```python
from build123d import *

# Parameters (mm, degrees)
PAD005_DEPTH           = 25
SKETCH014_W            = 3.1
SKETCH014_H            = 3.1
POCKET008_DEPTH        = 3.2
POCKET010_DEPTH        = 20.801
POCKET011_DEPTH        = 0.5
CHAMFER002_SIZE        = 0.5
SKETCH019_R            = 0.75
SKETCH019_R_2          = 1
POCKET012_DEPTH        = 25.001
CHAMFER003_SIZE        = 0.25
PAD009_DEPTH           = 1
CHAMFER_SIZE           = 0.5
PAD021_DEPTH           = 0.5
LINEARPATTERN001_COUNT = 4
LINEARPATTERN001_PITCH = 3.3333333333
SKETCH047_W            = 1.55
SKETCH047_H            = 10.5
PAD022_DEPTH           = 1
SKETCH048_W            = 1.5
SKETCH048_H            = 1.5
PAD023_DEPTH           = 4
SKETCH054_W            = 7.578003
SKETCH054_H            = 26.545825
POCKET038_DEPTH        = 8.751
POCKET038_DEPTH_BACK   = 8.751
FILLET005_R            = 0.5
SKETCH055_W            = 1.5
SKETCH055_H            = 1.5
POCKET039_DEPTH        = 2


with BuildPart() as part:
    # Sketch013 → Pad005 (new body)
    with BuildSketch(Plane.XY):
        with BuildLine():
            Line((-6.75, 4.75), (6.75, 4.75))
            ThreePointArc((8.75, 2.75), (8.1642135624, 4.1642135624), (6.75, 4.75))
            Line((8.75, 2.75), (8.75, -2.75))
            ThreePointArc((6.75, -4.75), (8.1642135624, -4.1642135624), (8.75, -2.75))
            Line((6.75, -4.75), (-6.75, -4.75))
            ThreePointArc((-8.75, -2.75), (-8.1642135624, -4.1642135624), (-6.75, -4.75))
            Line((-8.75, -2.75), (-8.75, 2.75))
            ThreePointArc((-6.75, 4.75), (-8.1642135624, 4.1642135624), (-8.75, 2.75))
        make_face()
    extrude(amount=-PAD005_DEPTH)

    # Sketch014 (on Face9 of Pad005) → Pocket008 (cut)
    with BuildSketch(Plane.XY):
        with Locations((6.15, 0)):
            Rectangle(SKETCH014_W, SKETCH014_H)
        with Locations((-6.15, 0)):
            Rectangle(SKETCH014_W, SKETCH014_H)
    extrude(amount=-POCKET008_DEPTH, mode=Mode.SUBTRACT)

    # Sketch017 → Pocket010 (cut, through all)
    with BuildSketch(Plane.XY.offset(-4.2)):
        with BuildLine():
            Line((-6.75, 3.75), (6.75, 3.75))
            ThreePointArc((7.75, 2.75), (7.4571067812, 3.4571067812), (6.75, 3.75))
            Line((7.75, 2.75), (7.75, -2.75))
            ThreePointArc((6.75, -3.75), (7.4571067812, -3.4571067812), (7.75, -2.75))
            Line((6.75, -3.75), (-6.75, -3.75))
            ThreePointArc((-7.75, -2.75), (-7.4571067812, -3.4571067812), (-6.75, -3.75))
            Line((-7.75, -2.75), (-7.75, 2.75))
            ThreePointArc((-6.75, 3.75), (-7.4571067812, 3.4571067812), (-7.75, 2.75))
        make_face()
    extrude(amount=-POCKET010_DEPTH, mode=Mode.SUBTRACT)

    # Sketch018 → Pocket011 (cut)
    with BuildSketch(Plane.XZ.offset(4.75)):
        with BuildLine():
            Line((1.0846232888, -1.5), (-1.0846232888, -1.5))
            ThreePointArc((-1.0846232888, -1.5), (-1.3011296398, -1.625), (-1.3011296398, -1.875))
            Line((-1.3011296398, -1.875), (-0.2165063509, -3.7536226433))
            ThreePointArc((-0.2165063509, -3.7536226433), (0, -3.8786226433), (0.2165063509, -3.7536226433))
            Line((0.2165063509, -3.7536226433), (1.3011296398, -1.875))
            ThreePointArc((1.3011296398, -1.875), (1.3011296398, -1.625), (1.0846232888, -1.5))
        make_face()
    extrude(amount=-POCKET011_DEPTH, mode=Mode.SUBTRACT)

    # Chamfer002
    chamfer002_edges = [part.edges().sort_by_distance(p)[0] for p in [
        (8.75, 0, 0),
    ]]
    chamfer(chamfer002_edges, length=CHAMFER002_SIZE)

    # Sketch019 (on Face8 of Chamfer002) → Pocket012 (cut, through all)
    with BuildSketch(Plane.XY):
        with Locations((0, -1.5)):
            Circle(SKETCH019_R)
        with Locations((2.9, -1.5)):
            Circle(SKETCH019_R)
        with Locations((-2.9, -1.5)):
            Circle(SKETCH019_R)
        with Locations((-6.1, 0)):
            Circle(SKETCH019_R_2)
        with Locations((6.1, 0)):
            Circle(SKETCH019_R_2)
    extrude(amount=-POCKET012_DEPTH, mode=Mode.SUBTRACT)

    # Chamfer003
    chamfer003_edges = [part.edges().sort_by_distance(p)[0] for p in [
        (-7.1, 0, -3.2),
        (5.1, 0, -3.2),
        (2.15, -1.5, 0),
        (-0.75, -1.5, 0),
        (-3.65, -1.5, 0),
    ]]
    chamfer(chamfer003_edges, length=CHAMFER003_SIZE)

    # Sketch027 → Pad009 (join)
    with BuildSketch(Plane.XY.offset(-25)):
        with BuildLine():
            Line((-6.75, 4.75), (6.75, 4.75))
            ThreePointArc((8.75, 2.75), (8.1642135624, 4.1642135624), (6.75, 4.75))
            Line((8.75, 2.75), (8.75, -2.75))
            ThreePointArc((6.75, -4.75), (8.1642135624, -4.1642135624), (8.75, -2.75))
            Line((6.75, -4.75), (-6.75, -4.75))
            ThreePointArc((-8.75, -2.75), (-8.1642135624, -4.1642135624), (-6.75, -4.75))
            Line((-8.75, -2.75), (-8.75, 2.75))
            ThreePointArc((-6.75, 4.75), (-8.1642135624, 4.1642135624), (-8.75, 2.75))
        make_face()
        with BuildLine():
            ThreePointArc((-5.45, 2.35), (-5.9096194078, 2.1596194078), (-6.1, 1.7))
            Line((-6.1, -1.7), (-6.1, 1.7))
            ThreePointArc((-6.1, -1.7), (-5.9096194078, -2.1596194078), (-5.45, -2.35))
            Line((5.45, -2.35), (-5.45, -2.35))
            ThreePointArc((5.45, -2.35), (5.9096194078, -2.1596194078), (6.1, -1.7))
            Line((6.1, 1.7), (6.1, -1.7))
            ThreePointArc((6.1, 1.7), (5.9096194078, 2.1596194078), (5.45, 2.35))
            Line((-5.45, 2.35), (5.45, 2.35))
        make_face(mode=Mode.SUBTRACT)
    extrude(amount=PAD009_DEPTH)

    # Chamfer
    chamfer_edges = [part.edges().sort_by_distance(p)[0] for p in [
        (0, -4.75, -25),
    ]]
    chamfer(chamfer_edges, length=CHAMFER_SIZE)

    # Sketch046 → Pad021 (join, symmetric)
    with BuildSketch(Plane.YZ.offset(5)):
        Polygon((3.75, -24), (3.75, -11.8), (0.05, -11.8), (0.05, -13.3), (2.45, -13.3), (2.45, -24), align=None)
    pad021 = extrude(amount=PAD021_DEPTH, both=True)

    # LinearPattern001: Pad021 ×4
    with Locations(*[(-i * LINEARPATTERN001_PITCH, 0, 0) for i in range(1, LINEARPATTERN001_COUNT)]):
        add(pad021)

    # Sketch047 → Pad022 (join, symmetric)
    with BuildSketch(Plane.XZ):
        with Locations((6.975, -18.75)):
            Rectangle(SKETCH047_W, SKETCH047_H)
    pad022 = extrude(amount=PAD022_DEPTH, both=True)

    # Mirrored008: Pad022 across Sketch047 V_Axis
    add(pad022.mirror(Plane(origin=(0, 0, 0), x_dir=(0, -1, 0), z_dir=(1, 0, 0))))

    # Sketch048 → Pad023 (join, symmetric)
    with BuildSketch(Plane.XZ):
        with Locations((7, -6.05)):
            Rectangle(SKETCH048_W, SKETCH048_H)
        with Locations((7, -12.55)):
            Rectangle(SKETCH048_W, SKETCH048_H)
    pad023 = extrude(amount=PAD023_DEPTH, both=True)

    # Mirrored009: Pad023 across Sketch048 V_Axis
    add(pad023.mirror(Plane(origin=(0, 0, 0), x_dir=(0, -1, 0), z_dir=(1, 0, 0))))

    # Sketch054 → Pocket038 (cut, two sides)
    with BuildSketch(Plane.YZ) as pocket038_sk:
        with Locations((-3.7890015, -17.4729125)):
            Rectangle(SKETCH054_W, SKETCH054_H)
    extrude(amount=-POCKET038_DEPTH, mode=Mode.SUBTRACT)
    extrude(pocket038_sk.sketch, amount=POCKET038_DEPTH_BACK, mode=Mode.SUBTRACT)

    # Fillet005
    fillet005_edges = [part.edges().sort_by_distance(p)[0] for p in [
        (-8.25, 0, -4.2),
        (8.25, 0, -4.2),
    ]]
    fillet(fillet005_edges, radius=FILLET005_R)

    # Sketch055 → Pocket039 (cut)
    with BuildSketch(Plane.XZ):
        with Locations((7, -6.05)):
            Rectangle(SKETCH055_W, SKETCH055_H)
        with Locations((7, -12.55)):
            Rectangle(SKETCH055_W, SKETCH055_H)
    pocket039 = extrude(amount=-POCKET039_DEPTH, mode=Mode.SUBTRACT)

    # Mirrored010: Pocket039 across Sketch055 V_Axis
    add(pocket039.mirror(Plane(origin=(0, 0, 0), x_dir=(0, -1, 0), z_dir=(1, 0, 0))), mode=Mode.SUBTRACT)


with BuildPart() as part_1:
    # Body012 placement: moved
    add(part.part.moved(Location((-18, 0, 0))))


solid = part_1.part
```
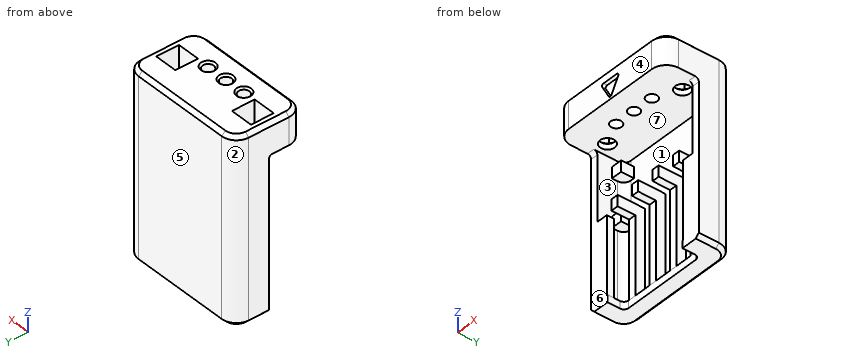
Can you work these out from the model? Positions are in its coordinate system, mm. Face numbers are marked on the shaded views. A direction names the side the tool comes from. Coordinates: 2 decimals unless noted, no trailing zeros. Write each loop counter-clockwise with the first axis right and the second up, starting at its lowest first coordinate (ties: lowest second). Pieces come first, ordered by that corner, then holes. Notation, with made-up numbers: M 38,-23 L 60,-23 A18 cw 60,0 Z; hole C 67.5,50 d6. An arc over 180 degrees is marked long. Answer as CSV lines item,"result".
Item 1: We'd pull the mould along X, two halves only. Please class the marked faces 1, 2, 3 and 4: +X half, -X half, draft (parallel to the pull), parting line (faces both ways), or undercut.
Geometry results:
face 1,"undercut"
face 2,"-X half"
face 3,"undercut"
face 4,"draft"
Item 2: Imagine slicing it at C-C on y = 0.5. State how many separate pieces and enclosed holes the cut face has, plus the area to 3 significant figures.
Geometry results:
separate pieces,"7"
enclosed holes,"0"
area,"133 mm2"
Item 3: On a 3-axis mill with a long thin cutter (end or side, diameter ignored), from which of +Z, -Z, +X, -X, +Y, -Y can I reach the whole of each face in a straight line? I mean the marked faces 5, 6 and 7. Say none if no direction works.
Geometry results:
face 5,"+Z, -Z, +X, -X, +Y"
face 6,"-Z, +X, -X, -Y"
face 7,"-Y"
Item 4: I'm going to push flat-ended pins straight in: P1, Ø3, axis at x = -16.5, z = -15, coming from the -Y side; P2, Ø5, axis at x = -18.5, y = -2.5, coming from the -Z side; P3, Ø3, axis at x = -10.5, z = -17.5, coming from the -Y side. Where does each tip first touch, or does it pass through?
Geometry results:
P1,"stops at y = 2.45"
P2,"stops at z = -4.2"
P3,"stops at y = 0"
Item 5: Please list where these lines run through material, in increasing order: line 1 along X through (y, z) = (0.25, -12); line 2 along Z through (x, y) = (-16.75, 3.5); line 3 along Z through (x, y) = (-19.5, 1.5).
Geometry results:
line 1,"x = -26.75 to -25.75, -23.5 to -22.5, -20.17 to -19.17, -16.83 to -15.83, -13.5 to -12.5, -10.25 to -9.25"
line 2,"z = -25 to -11.8, -4.2 to 0"
line 3,"z = -13.3 to -11.8, -4.2 to 0"
Item 6: Imagine slicing it at A-A on x = -20.9. List the corners of the cut face in (y, z) for me.
Geometry results:
outline,"M -4.75,-4.2 L -2.25,-4.2 L -2.25,-0.25 L -2.5,0 L -4.25,0 L -4.75,-0.5 Z; M -0.75,-4.2 L 3.75,-4.2 L 3.75,-24 L 2.35,-24 L 2.35,-25 L 4.25,-25 L 4.75,-24.5 L 4.75,-0.5 L 4.25,0 L -0.5,0 L -0.75,-0.25 Z"
